```python
from build123d import *

# Parameters (mm, degrees)
F0_W     = 2.7432
F0_H     = 15.24
F0_W_2   = 15.24
F0_H_2   = 2.7432
F1_DEPTH = 2.7432


# Not quite as in the source:
# - a feature names something its author has since deleted; it is built from what else it names


with BuildPart() as f1:
    # F0 (on Front) → F1 (new body)
    with BuildSketch(Plane.XZ):
        Polygon((-24.1134765283, 30.4756419325), (-87.1943765283, 30.4756419325), (-87.1943765283, -0.0043580675), (-87.1943765283, -15.2443580675), (-87.1943765283, -45.7243580675), (-24.1134765283, -45.7243580675), (-24.1134765283, -42.9811580675), (-8.8734765283, -42.9811580675), (-8.8734765283, -45.7243580675), (54.2074234717, -45.7243580675), (54.2074234717, -15.2443580675), (54.2074234717, -0.0043580675), (54.2074234717, 30.4756419325), (-8.8734765283, 30.4756419325), (-8.8734765283, 27.7324419325), (-24.1134765283, 27.7324419325), align=None)
        with Locations((-88.5659765283, -7.6243580675)):
            Rectangle(F0_W, F0_H)
        with Locations((55.5790234717, -7.6243580675)):
            Rectangle(F0_W, F0_H)
        with Locations((-16.4934765283, 29.1040419325)):
            Rectangle(F0_W_2, F0_H_2)
        with Locations((-16.4934765283, -44.3527580675)):
            Rectangle(F0_W_2, F0_H_2)
    extrude(amount=F1_DEPTH)


solid = f1.part
```
Could you check a few things on this model? Use its own coordinates, in mm. A direction names the side the tool comes from. Coordinates: 2 decimals unless noted, no trailing zeros. Loops run counter-clockwise (first coordinate to the right, second up) from the corner with the lowest first, then second, coordinate; pieces in that order, holes last.
1) Imagine slicing it at A-A (y = -2.2). List the corners of the cut face in (x, z) for me, and give its area (3 significant figures).
Reported:
outline: (-89.94, -15.24) - (-87.19, -15.24) - (-87.19, -45.72) - (54.21, -45.72) - (54.21, -15.24) - (56.95, -15.24) - (56.95, 0) - (54.21, 0) - (54.21, 30.48) - (-87.19, 30.48) - (-87.19, 0) - (-89.94, 0) - close
area: 10,900 mm2
2) Which directions (+Z, -Z, +X, -X, +Y, -Y) give clear straight access to the entire face, cutting with the end or side of a thin tool? Please do faces 1 (the face through (-87.194, -1, -30)), 2 (the face through (54.207, -1, -31)), 3 (the face through (-89, -1, -0.004)), 4 (the face through (56, -1, -0.004)), 5 (the face through (-17, -1, -45.724)).
Reported:
face 1: -Z, -X, +Y, -Y
face 2: -Z, +X, +Y, -Y
face 3: +Z, -X, +Y, -Y
face 4: +Z, +X, +Y, -Y
face 5: -Z, +X, -X, +Y, -Y
3) Please list where this line runs through material, in increasing order: line 1 along X through (y, z) = (-0.8, -37).
Reported:
line 1: x = -87.19 to 54.21
4) Will these pins go through, and if not, where does the flat tip stop? pin 1 Ø0.8 at (y, z) = (-2, 12) entering from +X; pin 2 Ø1 at (y, z) = (-1, -35.5) entering from -X; pin 3 Ø0.8 at (x, y) = (-88, -1.5) entering from -Z.
Reported:
pin 1: stops at x = 54.21
pin 2: stops at x = -87.19
pin 3: stops at z = -15.24
5) Imagine slicing it at B-B (z = 14). List the corners of the cut face in (x, y) for me.
Reported:
outline: (-87.19, -2.74) - (54.21, -2.74) - (54.21, 0) - (-87.19, 0) - close
